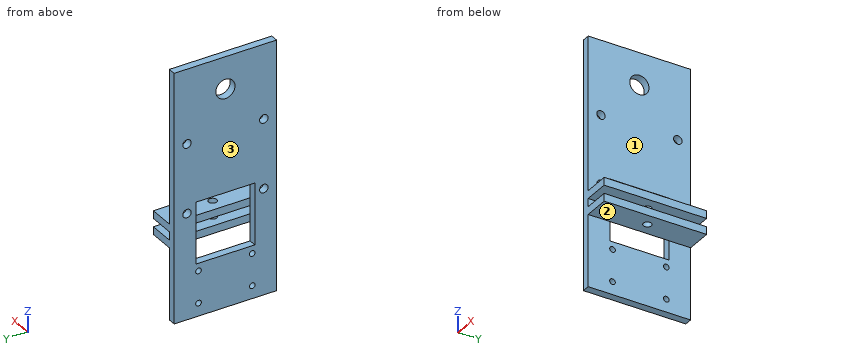
```python
from build123d import *

# Parameters (mm, degrees)
PAD_DEPTH       = 20
SKETCH001_R     = 1.6
POCKET_DEPTH    = 37.201
SKETCH002_R     = 1.1
SKETCH002_W     = 20
SKETCH002_H     = 23
POCKET001_DEPTH = 3.001
SKETCH003_R     = 1.65
SKETCH003_W     = 4
SKETCH003_H     = 23
POCKET002_DEPTH = 3.001
SKETCH004_W     = 25
SKETCH004_H     = 40
SKETCH004_R     = 3.75
PAD001_DEPTH    = 3


with BuildPart() as part:
    # Sketch → Pad (new body, symmetric)
    with BuildSketch(Plane.XZ):
        Polygon((-3, 39.6), (0, 39.6), (0, 4.6), (10, 4.6), (10, 1.6), (0, 1.6), (0, 0), (0, -1.6), (10, -1.6), (10, -4.6), (0, -4.6), (0, -32.6), (-3, -32.6), align=None)
    extrude(amount=PAD_DEPTH, both=True)

    # Sketch001 (on Face9 of Pad) → Pocket (cut, through all)
    with BuildSketch(Plane(origin=(0, 0, 4.6), x_dir=(-1, 0, 0), z_dir=(0, 0, 1))):
        with Locations((-5, 0)):
            Circle(SKETCH001_R)
    extrude(amount=-POCKET_DEPTH, mode=Mode.SUBTRACT)

    # Sketch002 (on Face13 of Pocket) → Pocket001 (cut, through all)
    with BuildSketch(Plane(origin=(0, 0, 0), x_dir=(0, 0, 1), z_dir=(1, 0, 0))):
        with Locations((-27.6, 10.5)):
            Circle(SKETCH002_R)
        with Locations((-15.1, 10.5)):
            Circle(SKETCH002_R)
        with Locations((-27.6, -10.5)):
            Circle(SKETCH002_R)
        with Locations((-15.1, -10.5)):
            Circle(SKETCH002_R)
        with Locations((-2.1, 0)):
            Rectangle(SKETCH002_W, SKETCH002_H)
    extrude(amount=-POCKET001_DEPTH, mode=Mode.SUBTRACT)

    # Sketch003 (on Face14 of Pocket001) → Pocket002 (cut, through all)
    with BuildSketch(Plane(origin=(0, 0, 0), x_dir=(0, 0, 1), z_dir=(1, 0, 0))):
        with Locations((8.6, 15)):
            Circle(SKETCH003_R)
        with Locations((35.6, 15)):
            Circle(SKETCH003_R)
        with Locations((35.6, -15)):
            Circle(SKETCH003_R)
        with Locations((8.6, -15)):
            Circle(SKETCH003_R)
        with Locations((9.9, 0)):
            Rectangle(SKETCH003_W, SKETCH003_H)
    extrude(amount=-POCKET002_DEPTH, mode=Mode.SUBTRACT)

    # Sketch004 (on Face12 of Pocket002) → Pad001 (join)
    with BuildSketch(Plane(origin=(0, 0, 0), x_dir=(0, 0, 1), z_dir=(1, 0, 0))):
        with Locations((52.1, 0)):
            Rectangle(SKETCH004_W, SKETCH004_H)
        with Locations((52.1, 0)):
            Circle(SKETCH004_R, mode=Mode.SUBTRACT)
    extrude(amount=-PAD001_DEPTH)


solid = part.part
```
Verification items for the finished model (mm, model axes). Face numbers are marked on the shaded views. A direction names the side the tool comes from. Round coordinates to 2 decimals unless told otherwise and drop trailing zeros. Order: outer loops, then holes, each group sorted by start corner. A loop starts at its lowest first (then second) coordinate and runs counter-clockwise, first axis right, second up. Notation, with made-up numbers: (-6.75, -12) -> (3.25, -12) arc R20 ccw to (3.25, -3) -> close; hole circle Ø8 at (78.25, -16). An arc over 180 degrees is marked (long way). Put each result on its own line as item: value. Start each with the question number.
(1) Section check D-D (y = 0). Enter the section's corners in (x, z).
(2) Depth check by flat-ended pin: pin 1 Ø2 at (y, z) = (15, 35.6) entering from -X; pin 2 Ø3.5 at (x, y) = (5, 0) entering from -Z; pin 3 Ø1.5 at (y, z) = (3, 2.5) entering from -X; pin 4 Ø2.5 at (y, z) = (-10.5, -27.6) entering from +X. Enter the tip coordinate at first touch or a pass-through.
(3) Material ranges on line 1 along Z through (x, y) = (-2.1, -10.5); line 2 along Y through (x, z) = (-0.9, -15.1); line 3 along Z through (x, y) = (-2.15, 15), recorded low to high.
(4) Tool access check on the marked faces 1, 2 and 3. Record the directions out of +Z, -Z, +X, -X, +Y, -Y that give a thin tool (end or side, any length) a straight path to the whole face; none if there is none.
(5) Section check B-B (z = 3.5). Enter the section's corners in (x, y).
(6) Section check C-C (x = 7.5). Enter the section's corners in (y, z), then the cut area to 3 significant figures.
(7) Section check A-A (y = 8.5). Enter the section's corners in (x, z), then the cut area to 3 significant figures.
Completed:
1. outline: (-3, -32.6) -> (0, -32.6) -> (0, -12.1) -> (-3, -12.1) -> close; (-3, 11.9) -> (0, 11.9) -> (0, 48.35) -> (-3, 48.35) -> close; (-3, 55.85) -> (0, 55.85) -> (0, 64.6) -> (-3, 64.6) -> close; (0, -4.6) -> (3.4, -4.6) -> (3.4, -1.6) -> (0, -1.6) -> close; (0, 1.6) -> (3.4, 1.6) -> (3.4, 4.6) -> (0, 4.6) -> close; (6.6, -4.6) -> (10, -4.6) -> (10, -1.6) -> (6.6, -1.6) -> close; (6.6, 1.6) -> (10, 1.6) -> (10, 4.6) -> (6.6, 4.6) -> close
2. pin 1: passes through
2. pin 2: stops at z = -4.6
2. pin 3: stops at x = 0
2. pin 4: stops at x = 0
3. line 1: z = -32.6 to -28.7, -26.5 to -16.2, -14 to -12.1, 11.9 to 64.6
3. line 2: y = -20 to -11.6, -9.4 to 9.4, 11.6 to 20
3. line 3: z = -32.6 to 6.95, 10.25 to 33.95, 37.25 to 64.6
4. face 1: +Z, +X, +Y, -Y
4. face 2: -Z, +X, +Y, -Y
4. face 3: +Z, -Z, -X, +Y, -Y
5. outline: (-3, -20) -> (10, -20) -> (10, 20) -> (-3, 20) -> (-3, 11.5) -> (0, 11.5) -> (0, -11.5) -> (-3, -11.5) -> close; hole circle Ø3.2 at (5, 0)
6. outline: (-20, -4.6) -> (20, -4.6) -> (20, -1.6) -> (-20, -1.6) -> close; (-20, 1.6) -> (20, 1.6) -> (20, 4.6) -> (-20, 4.6) -> close
6. area: 240 mm2
7. outline: (-3, -32.6) -> (0, -32.6) -> (0, -12.1) -> (-3, -12.1) -> close; (-3, 11.9) -> (0, 11.9) -> (0, 64.6) -> (-3, 64.6) -> close; (0, -4.6) -> (10, -4.6) -> (10, -1.6) -> (0, -1.6) -> close; (0, 1.6) -> (10, 1.6) -> (10, 4.6) -> (0, 4.6) -> close
7. area: 280 mm2
